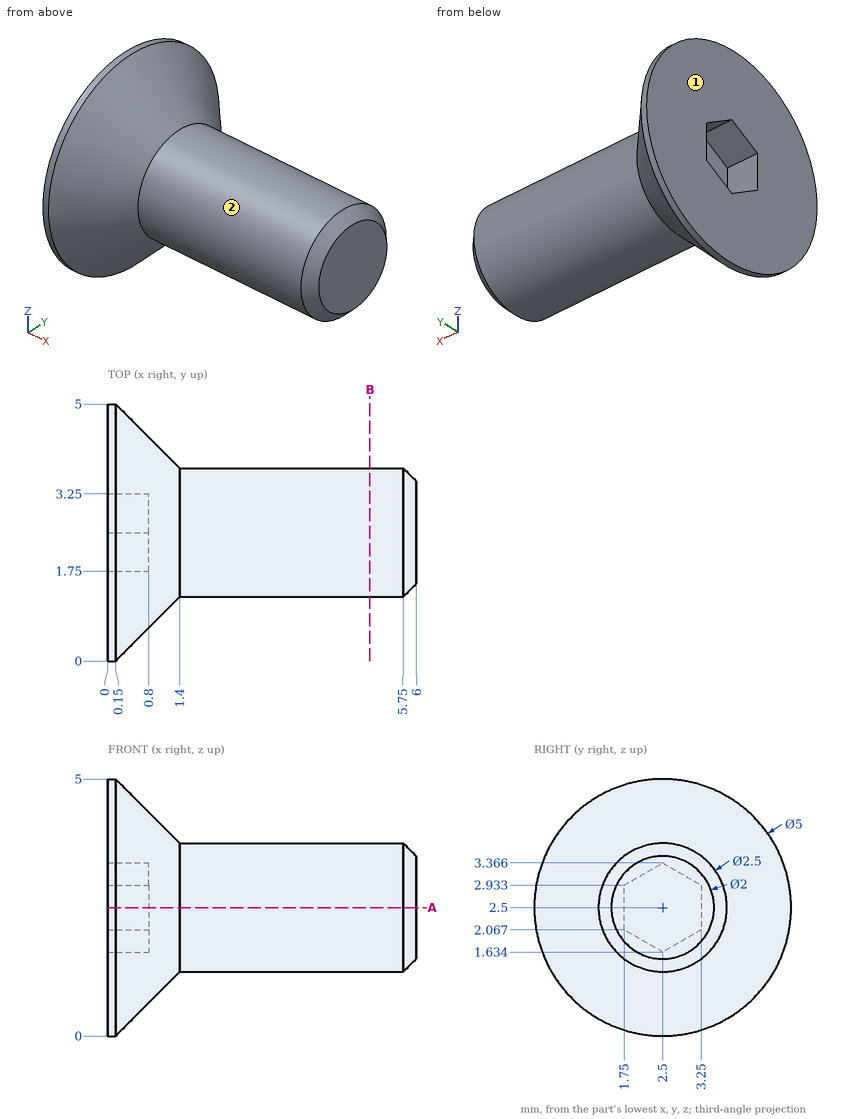
The drawing under review shows one solid part. Ordinate dimensions are in mm from its lowest x, y, z. A direction names the side the tool comes from. Give positions to 0.01 mm unless a question says otherwise; leave off trailing zeros. Order: outer loops, then holes, each group sorted by start corner. A loop starts at its lowest first (then second) coordinate and runs counter-clockwise, first axis right, second up. Notation, with made-up numbers: M 31,-1 L 63,-1 A19 cw 63,19 Z; hole C -14.75,79 d8. An arc over 180 degrees is marked long. One line per question, with ' | ' between items. Start each with the question number.
Q1. Machinability: for the marked faces 1 and 2, which of the approach directions +Z, -Z, +X, -X, +Y, -Y give a long, thin tool a straight path to every point of the face, cutting with its end or side? Answer none if there is none.
Q2. We need section B-B (x = 5.1). Write out the cut boundary in (y, z).
Q3. We need section A-A (z = 2.5). Write out the cut boundary in (x, y).
Q4. For L1, parallel to Z at x = 0.7, y = 1.8; L2, parallel to Z at x = 5.4, y = 2.95; L3, parallel to Y at x = 0.4, z = 3, list the stretches that pass through material, from the lowest coordinate up. Write a range as [from, to].
Q5. For pin 1 Ø1.5 at (x, y) = (5, 3.5) entering from +Z; pin 2 Ø0.6 at (x, z) = (0.5, 2.5) entering from -Y; pin 3 Ø1.2 at (y, z) = (3, 2) entering from -X; pin 4 Ø0.6 at (x, z) = (0.5, 2.5) entering from +Y, all flat-tipped, find the tip position at first contact; note any pin that passes through.
Returned:
1) face 1: +Z, -Z, -X, +Y, -Y | face 2: +X
2) outline: C 2.5,2.5 d2.5
3) outline: M 0,0 L 0.15,0 L 1.4,1.25 L 5.75,1.25 L 6,1.5 L 6,3.5 L 5.75,3.75 L 1.4,3.75 L 0.15,5 L 0,5 L 0,3.25 L 0.8,3.25 L 0.8,1.75 L 0,1.75 Z
4) L1: [0.68, 2.04], [2.96, 4.32] | L2: [1.33, 3.67] | L3: [0.31, 1.87], [3.13, 4.69]
5) pin 1: z = 3.72 | pin 2: y = 0.05 | pin 3: x = 0 | pin 4: y = 4.95
